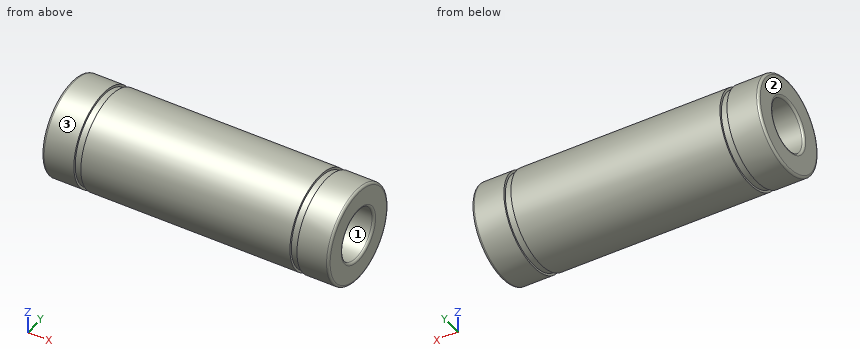
```python
from build123d import *


with BuildPart() as f1:
    # F0 (on Top) → F1 (revolve)
    with BuildSketch(Plane.XY):
        with BuildLine():
            Line((-17.5, 7.5), (-22.15, 7.5))
            ThreePointArc((-22.15, 7.5), (-22.397487, 7.397487), (-22.5, 7.15))
            Line((-22.5, 7.15), (-22.5, 4.35))
            ThreePointArc((-22.5, 4.35), (-22.397487, 4.102513), (-22.15, 4))
            Line((-22.15, 4), (22.15, 4))
            ThreePointArc((22.15, 4), (22.397487, 4.102513), (22.5, 4.35))
            Line((22.5, 4.35), (22.5, 7.15))
            ThreePointArc((22.5, 7.15), (22.397487, 7.397487), (22.15, 7.5))
            Line((22.15, 7.5), (17.5, 7.5))
            Line((17.5, 7.5), (17.5, 7.15))
            Line((17.5, 7.15), (16.4, 7.15))
            Line((16.4, 7.15), (16.4, 7.5))
            Line((16.4, 7.5), (-16.4, 7.5))
            Line((-16.4, 7.5), (-16.4, 7.15))
            Line((-16.4, 7.15), (-17.5, 7.15))
            Line((-17.5, 7.15), (-17.5, 7.5))
        make_face()
    revolve(axis=Axis((0, 0, 0), (1, 0, 0)))


solid = f1.part
```
Source: CAD feature listing. Evaluate the final solid. Frame: model axes, mm. Face numbers are marked on the shaded views. Coordinates: 2 decimals unless noted, no trailing zeros. Loops run counter-clockwise (first coordinate to the right, second up) from the corner with the lowest first, then second, coordinate; pieces in that order, holes last. Notation, with made-up numbers: M 39.25,55.25 L 75.25,55.25 A19 cw 75.25,65.25 Z; hole C 56.5,-8.75 d7. An arc over 180 degrees is marked long. Use a Markdown table: item, result. Add a question column.
Q1. First-contact query: pin 1 (3 mm diameter, centred on x = -16.5, z = -4.5, fed in from +Y); pin 2 (8 mm diameter, centred on x = -4, z = -1.5, fed in from +Y); pin 3 (1.5 mm diameter, centred on x = -15, z = -5, fed in from -Y). Flat tips, straight axial feed; report the tip coordinate or a pass-through.
Q2. Material intervals for L1, parallel to Z at x = -7, y = 0; L2, parallel to Y at x = -15.5, z = 2; L3, parallel to Y at x = -8.5, z = 0.5, sorted ascending.
Q3. Draft query along Y for the marked faces 1, 2 and 3. Return one class per face: pulls with the +Y half, pulls with the -Y half, needs draft (parallel to the pull), parting line crosses it, or undercut.
Q4. Section query C-C, the plane x = -11. Return loops of the section in (y, z), and give its area (3 significant figures).
Result:
| question | item | result |
|---|---|---|
| 1 | pin 1 | stops at y = 6.87 |
| 1 | pin 2 | stops at y = 7.5 |
| 1 | pin 3 | stops at y = -6.18 |
| 2 | L1 | z = -7.5 to -4, 4 to 7.5 |
| 2 | L2 | y = -7.23 to -3.46, 3.46 to 7.23 |
| 2 | L3 | y = -7.48 to -3.97, 3.97 to 7.48 |
| 3 | face 1 | undercut |
| 3 | face 2 | needs draft |
| 3 | face 3 | parting line crosses it |
| 4 | outline | C 0,0 d15; hole C 0,0 d8 |
| 4 | area | 126 mm2 |
